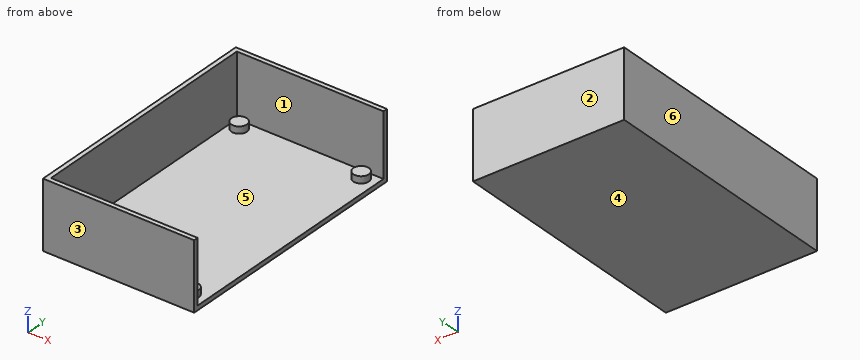
from build123d import *

# Parameters (mm, degrees)
SKETCH_W     = 67.25
SKETCH_H     = 110.8
PAD_DEPTH    = 30
THICKNESS_T  = -2
SKETCH001_R  = 3.45
PAD001_DEPTH = 3


with BuildPart() as part:
    # Sketch → Pad (new body)
    with BuildSketch(Plane.XY):
        with Locations((33.625, 55.4)):
            Rectangle(SKETCH_W, SKETCH_H)
    extrude(amount=PAD_DEPTH)

    # Thickness
    thickness_openings = [part.faces().sort_by_distance(p)[0] for p in [
        (33.625, 55.4, 30),
        (67.25, 55.4, 15),
    ]]
    offset(amount=THICKNESS_T, openings=thickness_openings)

    # Sketch001 (on Face9 of Thickness) → Pad001 (join)
    with BuildSketch(Plane.XY.offset(2)):
        with Locations((6.497925, 104.302401)):
            Circle(SKETCH001_R)
        with Locations((60.767925, 104.302401)):
            Circle(SKETCH001_R)
        with Locations((60.767925, 6.542401)):
            Circle(SKETCH001_R)
        with Locations((6.497925, 6.542401)):
            Circle(SKETCH001_R)
    extrude(amount=PAD001_DEPTH)


solid = part.part
Read the model definition and answer for the solid it produces. Units are mm, in the model's axes. Face numbers are marked on the shaded views. A direction names the side the tool comes from. Round coordinates to 2 decimals unless told otherwise and drop trailing zeros. Write each loop counter-clockwise with the first axis right and the second up, starting at its lowest first coordinate (ties: lowest second). Pieces come first, ordered by that corner, then holes.
1. The part is cut by section A-A, the plane x = 27.5. Determine the outline of the cut face in (y, z), then the cut area to 3 significant figures.
2. Straight lines are drawn through the part: L1, parallel to Y at x = 13, z = 21.25; L2, parallel to Y at x = 62.5, z = 3.25; L3, parallel to Z at x = 44, y = 26.5. For each, find the intervals that lie inside material, in ascending order.
3. The part is cut by section D-D, the plane z = 13. Determine the outline of the cut face in (x, y), then the cut area to 3 significant figures.
4. Determine the mould class of the marked faces 1, 2, 3 and 4 for opening direction Y: pulls with the +Y half, pulls with the -Y half, needs draft (parallel to the pull), parting line crosses it, or undercut.
5. Given pin 1 Ø8.5 at (y, z) = (76, 11.5) entering from +X; pin 2 Ø10 at (x, z) = (26, 19.5) entering from -Y; pin 3 Ø7.5 at (x, y) = (7, 8) entering from +Z; pin 4 Ø10 at (x, y) = (52, 22) entering from +Z, each flat-ended and moving along its own axis, determine where each tip first touches the part or whether it passes through.
6. The part is cut by section C-C, the plane y = 94. Determine the outline of the cut face in (x, z), then the cut area to 4 significant figures.
7. The part is cut by section B-B, the plane z = 3.5. Determine the outline of the cut face in (x, y).
8. Which of the six approach directions +Z, -Z, +X, -X, +Y, -Y give full straight-line access (tool end or side, diameter ignored) to the marked faces 5 and 6?
Values:
1. outline: (0, 0) - (110.8, 0) - (110.8, 30) - (108.8, 30) - (108.8, 2) - (2, 2) - (2, 30) - (0, 30) - close
1. area: 334 mm2
2. L1: y = 0 to 2, 108.8 to 110.8
2. L2: y = 0 to 2, 3.56 to 9.53, 101.32 to 107.29, 108.8 to 110.8
2. L3: z = 0 to 2
3. outline: (0, 0) - (67.25, 0) - (67.25, 2) - (2, 2) - (2, 108.8) - (67.25, 108.8) - (67.25, 110.8) - (0, 110.8) - close
3. area: 483 mm2
4. face 1: undercut
4. face 2: pulls with the +Y half
4. face 3: pulls with the -Y half
4. face 4: needs draft
5. pin 1: stops at x = 2
5. pin 2: stops at y = 0
5. pin 3: stops at z = 5
5. pin 4: stops at z = 2
6. outline: (0, 0) - (67.25, 0) - (67.25, 2) - (2, 2) - (2, 30) - (0, 30) - close
6. area: 190.5 mm2
7. outline: (0, 0) - (67.25, 0) - (67.25, 2) - (2, 2) - (2, 108.8) - (67.25, 108.8) - (67.25, 110.8) - (0, 110.8) - close; circle Ø6.9 at (6.5, 6.54); circle Ø6.9 at (6.5, 104.3); circle Ø6.9 at (60.77, 6.54); circle Ø6.9 at (60.77, 104.3)
8. face 5: +Z
8. face 6: +Z, -Z, -X, +Y, -Y
